The listing builds one solid part. Answer for the finished solid, in the listing's coordinates (mm). A direction names the side the tool comes from. Give positions to 0.01 mm unless a question says otherwise; leave off trailing zeros. Order: outer loops, then holes, each group sorted by start corner. A loop starts at its lowest first (then second) coordinate and runs counter-clockwise, first axis right, second up. Notation, with made-up numbers: (68, 2.25) - (127, 2.25) arc R35 cw to (127, 40.25) - close; hole circle Ø6 at (-19.5, 51). An arc over 180 degrees is marked (long way). Write each question's results on one line, items separated by ' | '. Start each with the question number.
1. Flat-ended cylindrical pins translate along their axes: pin 1 (10 mm diameter, centred on x = 13.5, z = 85.5, fed in from -Y); pin 2 (2 mm diameter, centred on y = -1.5, z = 79.5, fed in from +X). Find the tip coordinate at first contact, or state that the pin passes through.
2. Which of the six approach directions +Z, -Z, +X, -X, +Y, -Y give full straight-line access (tool end or side, diameter ignored) to faces 1 (the face through (106.243, 0.68, 124.463)), 2 (the face through (-0.295, 2.243, 34.121)), 3 (the face through (104, 0, 155.35))?
3. Find the intervals of material crossed by L1, parallel to Z at x = 45, y = -0.25; L2, parallel to X at y = 0.4, z = 103.5; L3, parallel to X at y = -0.25, z = 123, in increasing order.
4. Section A-A (z = 62.5) is taken. Give the vertices of the cut face in (x, y).
from build123d import *

# Parameters (mm, degrees)
F1_R = 2.262364


with BuildPart() as f2:
    # F2: sweep along a path in F0
    with BuildLine(Plane.XZ) as f2_path:
        Line((0, 0), (0, 67.300271))
        ThreePointArc((0, 67.300271), (3.719744, 76.280527), (12.7, 80.000271))
        Line((12.7, 80.000271), (91.384958, 80.000271))
        ThreePointArc((91.384958, 80.000271), (100.365214, 83.720015), (104.084958, 92.700271))
        Line((104.084958, 92.700271), (104.084958, 155.349578))
    # F1 (on Top) → F2 (sweep)
    with BuildSketch(Plane.XY):
        Circle(F1_R)
    sweep(path=f2_path.line)


solid = f2.part
Reported:
1) pin 1: y = -2.21 | pin 2: x = 99.44
2) face 1: +Z | face 2: -Z | face 3: +Z, +X, -X, +Y, -Y
3) L1: 77.75 to 82.25 | L2: 101.86 to 106.31 | L3: 101.84 to 106.33
4) outline: circle Ø4.52 at (0, 0)
